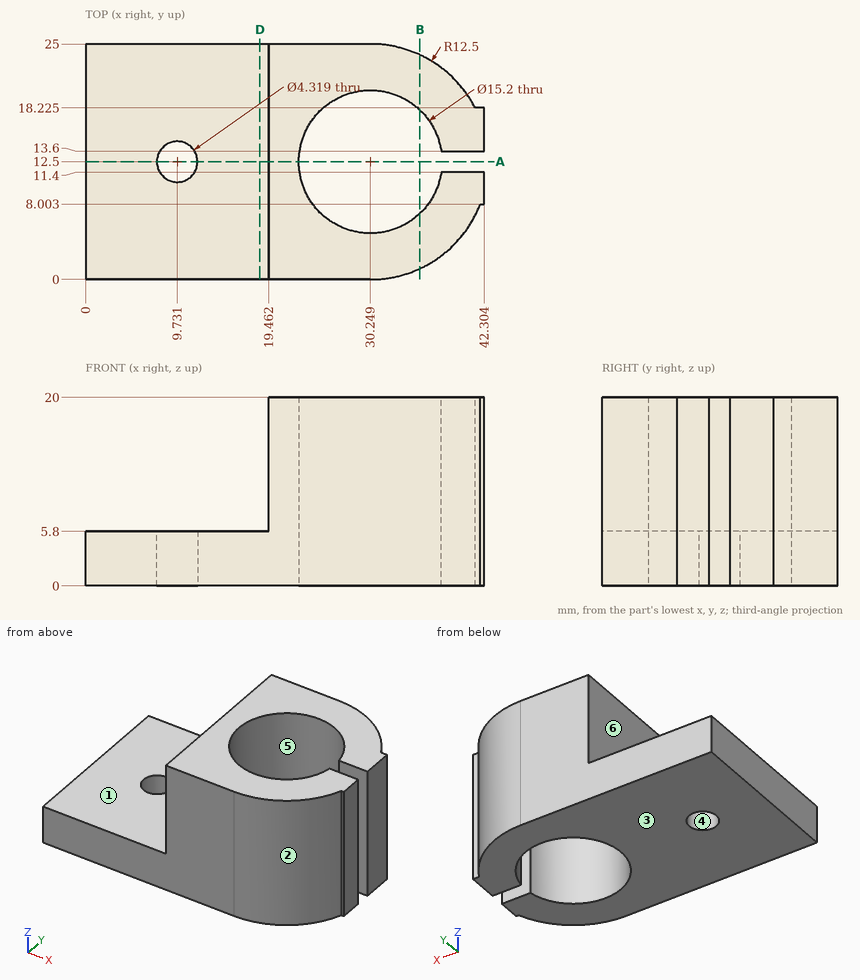
Print and shaded views of the part. All mm, measured from the part's lowest x, y and z. A direction names the side the tool comes from. Coordinates: 2 decimals unless noted, no trailing zeros. Write each loop counter-clockwise with the first axis right and the second up, starting at its lowest first coordinate (ties: lowest second). Pieces come first, ordered by that corner, then holes. Notation, with made-up numbers: (-13.75, 25) - (1.25, 25) arc R16 ccw to (1.25, 39) - close; hole circle Ø7 at (29.5, 86.25). An arc over 180 degrees is marked (long way). One line per question, with ' | ' between items. Start each with the question number.
Q1. Cut at B-B, the plane x = 35.5. List the corners of the cut face in (y, z).
Q2. Cut at A-A, the plane y = 12.5. List the corners of the cut face in (x, z).
Q3. Drill centre lines: line 1 (Y direction, x = 30.5, z = 10.75) (1 decimal); line 2 (Z direction, x = 9, y = 8); line 3 (Y direction, x = 25, z = 10) (1 decimal). Where is each one in solid material? Low to high. Write a range as [from, to].
Q4. 3-axis set-ups, long thin cutter, end or side, ignore diameter. For the marked faces 1 and 2: which of +Z, -Z, +X, -X, +Y, -Y reach the whole face in a straight line?
Q5. Pull direction X, two halves, no side cores. Call the marked faces 3, 4, 5 and 6: pulls with the +X half, pulls with the -X half, needs draft (parallel to the pull), parting line crosses it, or undercut.
Q6. Pin check, flat tips, straight feed: pin 1 (1 mm diameter, centred on x = 41.5, z = 13.5, fed in from +Y) (1 decimal); pin 2 (4 mm diameter, centred on y = 2.5, z = 18, fed in from -X); pin 3 (1.4 mm diameter, centred on x = 39, z = 13.5, fed in from +Y). Stop position of each tip, or through.
Q7. Cut at D-D, the plane x = 18.5. List the corners of the cut face in (y, z), then the cut area to 3 significant figures.
Answer below:
1) outline: (1.16, 0) - (7.01, 0) - (7.01, 20) - (1.16, 20) - close; (17.99, 0) - (23.84, 0) - (23.84, 20) - (17.99, 20) - close
2) outline: (0, 0) - (7.57, 0) - (7.57, 5.8) - (0, 5.8) - close; (11.89, 0) - (22.65, 0) - (22.65, 20) - (19.46, 20) - (19.46, 5.8) - (11.89, 5.8) - close
3) line 1: [0, 4.9], [20.1, 25] | line 2: [0, 5.8] | line 3: [0, 7], [18, 25]
4) face 1: +Z, -X, +Y, -Y | face 2: +Z, -Z, +X, -Y
5) face 3: needs draft | face 4: undercut | face 5: undercut | face 6: pulls with the -X half
6) pin 1: y = 18.9 | pin 2: x = 19.46 | pin 3: y = 22.06
7) outline: (0, 0) - (25, 0) - (25, 5.8) - (0, 5.8) - close | area: 145 mm^2
